Autodesk Fusion 360 part; units mm, degrees
sketch "Sketch1" plane through (0, 0, 0) normal (0, 0, 1) x (1, 0, 0)
  line L0 (-32.7972, 24.5979) -> (36.9278, 24.5979)
  line L1 (36.9278, 24.5979) -> (36.9278, -20.9771)
  line L2 (36.9278, -20.9771) -> (-32.7972, -20.9771)
  line L3 (-32.7972, -20.9771) -> (-32.7972, 24.5979)
  line L4 (-42.2972, 34.0979) -> (46.4278, 34.0979)
  line L5 (46.4278, 34.0979) -> (46.4278, -30.4771)
  line L6 (46.4278, -30.4771) -> (-42.2972, -30.4771)
  line L7 (-42.2972, -30.4771) -> (-42.2972, 34.0979)
  circle A0 centre (-37.2972, 29.0979) radius 1.7
  circle A1 centre (-37.2972, 29.0979) radius 3
  circle A2 centre (41.4278, 29.0979) radius 1.7
  circle A3 centre (41.4278, 29.0979) radius 3
  circle A4 centre (41.4278, -25.4771) radius 1.7
  circle A5 centre (41.4278, -25.4771) radius 3
  circle A6 centre (-37.2972, -25.4771) radius 1.7
  circle A7 centre (-37.2972, -25.4771) radius 3
  dimension "d14" = 6
  dimension "d18" = 6
  dimension "d22" = 6
extrude "Extrude1" add sketch "Sketch1" along normal blind 9.9 from surface at 3.1 contours A1 | A3 | A5 | A7 makes body 1 at (44.424, 28.9484, 9.7) makes body 2 at (-34.301, -25.6266, 9.7) makes body 3 at (-34.301, 28.9484, 9.7) makes body 4 at (44.424, -25.6266, 9.7)
extrude "Extrude2" add sketch "Sketch1" along normal blind 13 contours L4 L5 L6 L7 bodies 1 2 3 4
extrude "Extrude3" add sketch "Sketch1" along normal blind 3 contours L0 L1 L2 L3 bodies 1
sketch "Sketch2" plane through (0, 0, 13) normal (0, 0, 1) x (-1, 0, 0)
  circle A0 centre (-41.4278, -29.0979) radius 1.7
  circle A1 centre (-41.4278, 25.4771) radius 1.7
  line L0 (-36.9278, 20.9771) -> (32.7972, 20.9771)
  line L1 (32.7972, 20.9771) -> (32.7972, -24.5979)
  line L2 (32.7972, -24.5979) -> (-36.9278, -24.5979)
  line L3 (-36.9278, -24.5979) -> (-36.9278, 20.9771)
  line L4 (42.2972, 30.4771) -> (-46.4278, 30.4771)
  line L5 (-46.4278, 30.4771) -> (-46.4278, -34.0979)
  line L6 (-46.4278, -34.0979) -> (42.2972, -34.0979)
  line L7 (42.2972, -34.0979) -> (42.2972, 30.4771)
  circle A2 centre (37.2972, 25.4771) radius 1.7
  circle A3 centre (37.2972, -29.0979) radius 1.7
  line L8 (-12.3028, -34.0979) -> (-30.8028, -34.0979)
  line L9 (-30.8028, -34.0979) -> (-30.8028, -24.5979)
  line L10 (-30.8028, -24.5979) -> (-12.3028, -24.5979)
  line L11 (-12.3028, -24.5979) -> (-12.3028, -34.0979)
  line L12 (42.2972, 30.4771) -> (42.2972, -34.0979)
  dimension "d30" = 18.5
  dimension "d31" = 54.6
extrude "Extrude4" cut sketch "Sketch2" against normal blind 7.5 contours L2 L6 L8 L9 L10 L11 bodies 1
fillet "Fillet1" radius 5 4 edges at (-42.2972, -30.4771, 6.5) (-42.2972, 34.0979, 6.5) (46.4278, -30.4771, 6.5) (46.4278, 34.0979, 6.5) on bodies 1
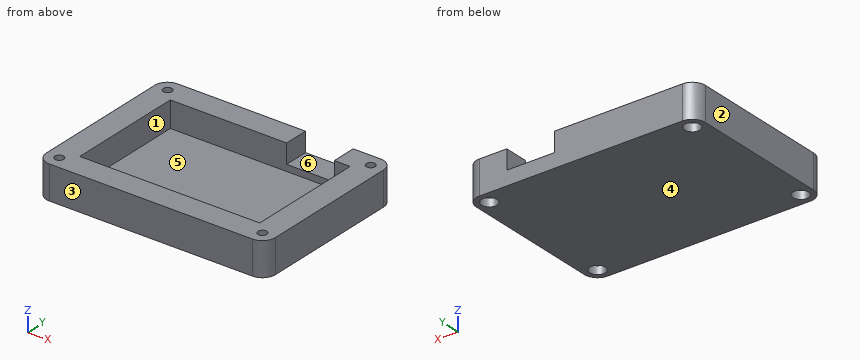
Model file for the job. Use its own axes, mm. Face numbers are marked on the shaded views. A direction names the side the tool comes from. Round coordinates to 2 decimals unless told otherwise and drop trailing zeros. Order: outer loops, then holes, each group sorted by start corner. A loop starts at its lowest first (then second) coordinate and runs counter-clockwise, first axis right, second up.
(1) Band-saw the part on D-D (z = 10.5). List the corners of the cut face in (x, y).
(2) Band-saw the part on A-A (z = 1.5). List the corners of the cut face in (x, y), then the cut area to 3 significant figures.
(3) Pin check, flat tips, straight feed: pin 1 (1.8 mm diameter, centred on x = -38.5, y = 29, fed in from -Z); pin 2 (12 mm diameter, centred on x = 25.5, y = 21.5, fed in from -Z); pin 3 (7.5 mm diameter, centred on x = 19, y = 28, fed in from +Z); pin 4 (4 mm diameter, centred on x = 13, y = 11.5, fed in from +Z). Stop position of each tip, or through.
(4) Band-saw the part on C-C (y = 10.5). List the corners of the cut face in (x, z).
(5) Pull direction X, two halves, no side cores. Call the marked faces 1, 2 and 3: released by +X, released by -X, zero draft, split by the parting line, or undercut.
(6) Drill centre lines: line 1 (X direction, y = 23, z = 11.5); line 2 (X direction, y = 30, z = 3.75); line 3 (Y direction, x = -2, z = 8.5). Where is each one in solid material? Low to high.
(7) Band-saw the part on B-B (x = 18). List the corners of the cut face in (y, z).
(8) 3-axis set-ups, long thin cutter, end or side, ignore diameter. For the marked faces 4, 5 and 6: which of +Z, -Z, +X, -X, +Y, -Y reach the whole face in a straight line?
Verdict:
1. outline: (-42.3, -25.48) arc R5 ccw to (-37.3, -30.48) - (41.43, -30.48) arc R5 ccw to (46.43, -25.48) - (46.43, 29.1) arc R5 ccw to (41.43, 34.1) - (30.8, 34.1) - (30.8, 24.6) - (36.93, 24.6) - (36.93, -20.98) - (-32.8, -20.98) - (-32.8, 24.6) - (12.3, 24.6) - (12.3, 34.1) - (-37.3, 34.1) arc R5 ccw to (-42.3, 29.1) - close; hole circle Ø3.4 at (-37.3, -25.48); hole circle Ø3.4 at (-37.3, 29.1); hole circle Ø3.4 at (41.43, -25.48); hole circle Ø3.4 at (41.43, 29.1)
2. outline: (-42.3, -25.48) arc R5 ccw to (-37.3, -30.48) - (41.43, -30.48) arc R5 ccw to (46.43, -25.48) - (46.43, 29.1) arc R5 ccw to (41.43, 34.1) - (-37.3, 34.1) arc R5 ccw to (-42.3, 29.1) - close; hole circle Ø6 at (-37.3, -25.48); hole circle Ø6 at (-37.3, 29.1); hole circle Ø6 at (41.43, -25.48); hole circle Ø6 at (41.43, 29.1)
2. area: 5,590 mm2
3. pin 1: stops at z = 3.1
3. pin 2: stops at z = 0
3. pin 3: stops at z = 5.5
3. pin 4: stops at z = 3
4. outline: (-42.3, 0) - (46.43, 0) - (46.43, 13) - (36.93, 13) - (36.93, 3) - (-32.8, 3) - (-32.8, 13) - (-42.3, 13) - close
5. face 1: undercut
5. face 2: released by -X
5. face 3: zero draft
6. line 1: x = -42.3 to -32.8, 36.93 to 46.43
6. line 2: x = -42.22 to -38.74, -35.86 to 39.99, 42.87 to 46.35
6. line 3: y = -30.48 to -20.98, 24.6 to 34.1
7. outline: (-30.48, 0) - (34.1, 0) - (34.1, 5.5) - (24.6, 5.5) - (24.6, 3) - (-20.98, 3) - (-20.98, 13) - (-30.48, 13) - close
8. face 4: -Z, +X, -X, +Y, -Y
8. face 5: +Z
8. face 6: +Z, +Y
